Geometry check sheet. Reference: the model listing, model coordinates, mm. Round coordinates to 2 decimals unless told otherwise and drop trailing zeros. Loops run counter-clockwise (first coordinate to the right, second up) from the corner with the lowest first, then second, coordinate; pieces in that order, holes last. Notation, with made-up numbers: M 30,71 L 80,71 A8 ccw 80,81 Z; hole C 48.25,38 d9. An arc over 180 degrees is marked long. Write item = value, one per line.
from build123d import *

# Parameters (mm, degrees)
SKETCH1_W           = 40.64
SKETCH1_H           = 177.8
BOSS_EXTRUDE1_DEPTH = 3.048
SKETCH2_R           = 2.0066
CUT_EXTRUDE1_DEPTH  = 3.048
SKETCH3_R           = 2.0193
CUT_EXTRUDE2_DEPTH  = 92.243644732
FILLET1_R           = 6.35


with BuildPart() as part:
    # Sketch1 → Boss-Extrude1 (new body)
    with BuildSketch(Plane.XY):
        Rectangle(SKETCH1_W, SKETCH1_H)
    extrude(amount=BOSS_EXTRUDE1_DEPTH)

    # Sketch2 → Cut-Extrude1 (cut)
    with BuildSketch(Plane.XY.offset(3.048)):
        with Locations((0, -76.2)):
            Circle(SKETCH2_R)
        with Locations((0, 82.55)):
            Circle(SKETCH2_R)
        with Locations((0, 76.2)):
            Circle(SKETCH2_R)
        with Locations((0, 69.85)):
            Circle(SKETCH2_R)
        with Locations((0, 63.5)):
            Circle(SKETCH2_R)
        with Locations((16.002, -76.2)):
            Circle(SKETCH2_R)
        with Locations((-16.002, -76.2)):
            Circle(SKETCH2_R)
    extrude(amount=-CUT_EXTRUDE1_DEPTH, mode=Mode.SUBTRACT)

    # Sketch3 → Cut-Extrude2 (cut, through all)
    with BuildSketch(Plane.XY.offset(3.048)):
        with Locations((0, -16.4846)):
            Circle(SKETCH3_R)
        with Locations((0, -10.1346)):
            Circle(SKETCH3_R)
        with Locations((0, -3.7846)):
            Circle(SKETCH3_R)
        with Locations((0, 2.5654)):
            Circle(SKETCH3_R)
        with Locations((0, 8.9154)):
            Circle(SKETCH3_R)
        with Locations((0, 15.2654)):
            Circle(SKETCH3_R)
        with Locations((0, 21.6154)):
            Circle(SKETCH3_R)
        with Locations((0, 27.9654)):
            Circle(SKETCH3_R)
        with Locations((0, 34.3154)):
            Circle(SKETCH3_R)
        with Locations((0, 40.6654)):
            Circle(SKETCH3_R)
    extrude(amount=-CUT_EXTRUDE2_DEPTH, mode=Mode.SUBTRACT)

    # Fillet1
    fillet1_edges = [part.edges().sort_by_distance(p)[0] for p in [
        (20.32, -88.9, 1.524),
        (-20.32, -88.9, 1.524),
        (-20.32, 88.9, 1.524),
        (20.32, 88.9, 1.524),
    ]]
    fillet(fillet1_edges, radius=FILLET1_R)


solid = part.part
(1) Sectioned sample at C-C on y = 63.5. Record the cut outline in (x, z).
Result set:
outline = M -20.32,0 L -2.01,0 L -2.01,3.05 L -20.32,3.05 Z; M 2.01,0 L 20.32,0 L 20.32,3.05 L 2.01,3.05 Z
(2) Release check for a two-part mould opening along Y. For faces 1 (the cylindrical face through (-18.5, -87, 1.5)), 2 (the cylindrical face through (-0.26, 71.84, 1.55)), 3 (the flat face through (20.32, -1, 2)) record: released by +Y, released by -Y, zero draft, split by the parting line, or undercut.
Result set:
face_1 = released by -Y
face_2 = undercut
face_3 = zero draft
(3) Sectioned sample at A-A on y = -76.2. Record the cut outline in (x, z).
Result set:
outline = M -20.32,0 L -18.01,0 L -18.01,3.05 L -20.32,3.05 Z; M -14,0 L -2.01,0 L -2.01,3.05 L -14,3.05 Z; M 2.01,0 L 14,0 L 14,3.05 L 2.01,3.05 Z; M 18.01,0 L 20.32,0 L 20.32,3.05 L 18.01,3.05 Z
(4) Material ranges on line 1 along Y through (x, z) = (-15.5, 1.3); line 2 along X through (y, z) = (35, 0.85), recorded low to high. Write a range as from..to.
Result set:
line_1 = -88.71..-78.14, -74.26..88.71
line_2 = -20.32..-1.9, 1.9..20.32
(5) Sectioned sample at B-B on z = 1.6. State how many separate pieces and enclosed holes the cut face has, then the cut area to 3 significant figures.
Result set:
separate_pieces = 1
enclosed_holes = 17
area = 6,970 mm2
